Autodesk Inventor part; units mm, degrees
ref_plane "YZ Plane" through (0, 0, 0) normal (1, 0, 0) x (0, 1, 0)
ref_plane "XZ Plane" through (0, 0, 0) normal (0, 1, 0) x (-1, 0, 0)
ref_plane "XY Plane" through (0, 0, 0) normal (0, 0, 1) x (1, 0, 0)
sketch "Эскиз8" plane through (0, 0, 0) normal (1, 0, 0) x (0, 1, 0)
  line L0 (0, 0) -> (10.4, 0)
  line L1 (10.4, 0) -> (10.4, -10.4)
  line L2 (10.4, -10.4) -> (0, -10.4)
  line L3 (0, -10.4) -> (0, 0)
  line L4 (5.2, 0) -> (5.2, 4)
  line L5 (5.2, -10.4) -> (5.2, -14.4)
  circle A0 centre (5.2, 4) radius 1.6
  circle A1 centre (5.2, -14.4) radius 1.6
  line L6 (5.2, 4) -> (7.9, 4)
  line L7 (7.9, 2.4412) -> (5.2, 0.8823)
  line L8 (5.2, 0.8823) -> (2.5, 2.4412)
  line L9 (2.5, 2.4412) -> (2.5, 5.5588)
  line L10 (2.5, 5.5588) -> (5.2, 7.1177)
  line L11 (5.2, 7.1177) -> (7.9, 5.5588)
  line L12 (7.9, 5.5588) -> (7.9, 2.4412)
  line L13 (7.9, -15.9588) -> (5.2, -17.5177)
  line L14 (5.2, -17.5177) -> (2.5, -15.9588)
  line L15 (2.5, -15.9588) -> (2.5, -12.8412)
  line L16 (2.5, -12.8412) -> (5.2, -11.2823)
  line L17 (5.2, -11.2823) -> (7.9, -12.8412)
  line L18 (7.9, -12.8412) -> (7.9, -15.9588)
  circle A2 centre (5.2, 4) radius 5.2
  circle A3 centre (5.2, -14.4) radius 5.2
  line L19 (10.4, 4) -> (10.4, 0)
  line L20 (10.4, -10.4) -> (10.4, -14.4)
  line L21 (0, -14.4) -> (0, -10.4)
  line L22 (0, 4) -> (0, 0)
  line L23 (7.9, 5.5588) -> (7.9, 8.4441)
  line L24 (2.5, 5.5588) -> (2.5, 8.4441)
  line L25 (2.5, -15.9588) -> (2.5, -18.8441)
  line L26 (7.9, -15.9588) -> (7.9, -18.8441)
  line L27 (0, 0) -> (-3, 0)
  line L28 (-3, 0) -> (-3, -10.4)
  line L29 (-3, -10.4) -> (0, -10.4)
  line L30 (0, -10.4) -> (0, 0)
  line L31 (10.4, 0) -> (8.9, 2.5981)
  line L32 (10.4, -10.4) -> (8.9, -12.9981)
  line L33 (10.4, -10.4) -> (13.4, -10.4) construction
  line L34 (8.9, -12.9981) -> (4.4, -10.4)
  line L35 (8.9, 2.5981) -> (4.4, 0)
  line L36 (-3, 0) -> (0.663, 6.5408)
  line L37 (-3, -10.4) -> (0.663, -16.9408)
  line L38 (10.4, 0) -> (12.9981, 1.5)
  line L39 (12.9981, 1.5) -> (9.5707, 6.8173)
  line L40 (10.4, -10.4) -> (12.9981, -11.9)
  line L41 (12.9981, -11.9) -> (9.5707, -17.2173)
  point P0 (7.9, -14.4)
  dimension "d51" = 10.4
  dimension "d52" = 10.4
  dimension "d53" = 4
  dimension "d54" = 4
  dimension "d55" = 3.2
  dimension "d56" = 3.2
  dimension "d57" = 2.7
  dimension "d58" = 3
  dimension "d59" = 3
  dimension "d60" = 3
  dimension "d61" = 120
  dimension "d62" = 3
  dimension "d63" = 3
extrude "Выдавливание6" add sketch "Эскиз8" along normal blind 5 contours L0 A2 L24 L9 L8 L4 L35 | L0 L22 A2 | L4 L7 L12 L23 A2 L31 L35 | L27 L36 A2 L22 | L3 L29 L28 L27 | L31 A2 L19 | L19 A2 L39 L38 | L2 A3 L21 | L21 A3 L37 L29 | L40 L41 A3 L20 | L20 A3 L32 | L2 L34 L5 L16 L15 L25 A3 | A3 L26 L18 L17 L5 L34 L32
sketch "Эскиз9" plane through (0, 0, 0) normal (-1, 0, 0) x (0, 0, 1)
  arc A0 (-18.8441, 2.5) -> (-16.9408, 0.663) centre (-14.4, 5.2) ccw
  circle A1 centre (-14.4, 5.2) radius 5.2
  circle A2 centre (-14.4, 5.2) radius 1.6
  arc A3 (6.5408, 0.663) -> (8.4441, 2.5) centre (4, 5.2) ccw
  circle A4 centre (4, 5.2) radius 5.2
  circle A5 centre (4, 5.2) radius 1.6
  line L0 (2.5981, 8.9) -> (0, 10.4)
  line L1 (0, 10.4) -> (2.5981, 8.9)
  line L2 (0, 4.4) -> (2.5981, 8.9)
  line L3 (2.5981, 8.9) -> (0, 4.4)
  line L4 (0, 0) -> (0, 4.4)
  line L5 (0, 4.4) -> (0, 0)
  line L6 (-10.4, 4.4) -> (-10.4, 0)
  line L7 (0, 0) -> (-10.4, 0)
  line L8 (-10.4, 0) -> (-10.4, 1.8774)
  line L9 (-10.4, 10.4) -> (-12.9981, 8.9)
  line L10 (-11.699, 9.65) -> (-10.4, 10.4)
  line L11 (-11.9, 12.9981) -> (-10.4, 10.4)
  line L12 (-10.4, 10.4) -> (-11.9, 12.9981)
  line L13 (-17.2173, 9.5707) -> (-11.9, 12.9981)
  line L14 (-11.9, 12.9981) -> (-17.2173, 9.5707)
  line L15 (0, 10.4) -> (1.5, 12.9981)
  line L16 (0, 10.4) -> (1.5, 12.9981)
  line L17 (1.5, 12.9981) -> (6.8173, 9.5707)
  line L18 (1.5, 12.9981) -> (6.8173, 9.5707)
  line L19 (0, -3) -> (-10.4, -3)
  line L20 (0, -3) -> (6.5408, 0.663)
  line L21 (6.5408, 0.663) -> (0, -3)
  line L22 (-10.4, -3) -> (-16.9408, 0.663)
  line L23 (-10.4, -3) -> (-16.9408, 0.663)
  line L24 (-10.4, -3) -> (0, -3)
  line L25 (-10.4, 0) -> (0, 0)
  line L26 (0, 0) -> (-10.4, 0)
  line L27 (-10.4, 0) -> (-10.4, 1.8774)
  line L28 (0, 1.8774) -> (0, 0)
  line L29 (-11.699, 9.65) -> (-12.9981, 8.9)
  line L30 (-12.9981, 8.9) -> (-10.4, 4.4)
  line L31 (-10.4, 4.4) -> (-12.9981, 8.9)
  line L32 (-12.9981, 8.9) -> (-10.4, 4.4)
  line L33 (-10.4, 4.4) -> (-10.4, 1.8774)
  line L34 (0, 1.8774) -> (0, 4.4)
  line L35 (2.5981, 8.9) -> (0, 4.4)
  line L36 (1.299, 9.65) -> (2.5981, 8.9)
  point P0 (-18.8441, 2.5)
  point P1 (-16.9408, 0.663)
  point P2 (6.5408, 0.663)
  point P3 (8.4441, 2.5)
  dimension "d66" = 3.2
  dimension "d67" = 3.2
extrude "Выдавливание7" add sketch "Эскиз9" along normal blind 5 contours A1 L9 L30 L6 A0 | A1 L6 L7 L4 A4 L20 L19 L22 | L13 L11 L9 A1 | A4 L4 L2 L0 A3 | L0 L15 L17 A4
sketch "Эскиз10" plane through (5, 0, 0) normal (1, 0, 0) x (0, 0, -1)
  line L0 (-1.5, 12.9981) -> (-6.8173, 9.5707)
  line L1 (0, 10.4) -> (-1.5, 12.9981)
  line L2 (-1.5, 12.9981) -> (0, 10.4)
  line L3 (-2.5981, 8.9) -> (0, 10.4)
  line L4 (0, 10.4) -> (-2.5981, 8.9)
  line L5 (0, 4.4) -> (-2.5981, 8.9)
  line L6 (-2.5981, 8.9) -> (0, 4.4)
  line L7 (0, 0) -> (0, 4.4)
  line L8 (0, 4.4) -> (0, 0)
  line L9 (10.4, 0) -> (0, 0)
  line L10 (0, 0) -> (10.4, 0)
  line L11 (10.4, 4.4) -> (10.4, 0)
  line L12 (10.4, 0) -> (10.4, 4.4)
  line L13 (10.4, 10.4) -> (12.9981, 8.9)
  line L14 (10.4, 4.4) -> (12.9981, 8.9)
  line L15 (12.9981, 8.9) -> (10.4, 10.4)
  line L16 (11.9, 12.9981) -> (10.4, 10.4)
  line L17 (10.4, 10.4) -> (11.9, 12.9981)
  line L18 (17.2173, 9.5707) -> (11.9, 12.9981)
  line L19 (11.9, 12.9981) -> (17.2173, 9.5707)
  line L20 (17.2173, 9.5707) -> (13.6704, -1.1685)
  line L21 (10.4, -3) -> (16.9408, 0.663)
  line L22 (10.4, -3) -> (13.6704, -1.1685)
  line L23 (0, -3) -> (10.4, -3)
  line L24 (-6.5408, 0.663) -> (0, -3)
  line L25 (10.4, -3) -> (0, -3)
  arc A0 (-8.4441, 2.5) -> (-6.5408, 0.663) centre (-4, 5.2) ccw
  line L26 (0, -3) -> (-6.5408, 0.663)
  line L27 (-3.2704, -1.1685) -> (-6.8173, 9.5707)
  line L28 (-6.8173, 9.5707) -> (-1.5, 12.9981)
extrude "Выдавливание8" add sketch "Эскиз10" along normal blind 157.53
sketch "Эскиз13" plane through (162.53, 0, 0) normal (1, 0, 0) x (0, 0, -1)
  line L0 (-6.8173, 9.5707) -> (-1.5, 12.9981)
  line L1 (-1.5, 12.9981) -> (-6.8173, 9.5707)
  line L2 (-6.5408, 0.663) -> (-3.2704, -1.1685)
  line L3 (-6.8173, 9.5707) -> (-3.2704, -1.1685)
  line L4 (-3.2704, -1.1685) -> (0, -3)
  line L5 (10.4, -3) -> (0, -3)
  line L6 (0, -3) -> (10.4, -3)
  line L7 (16.9408, 0.663) -> (10.4, -3)
  line L8 (10.4, -3) -> (13.6704, -1.1685)
  line L9 (13.6704, -1.1685) -> (17.2173, 9.5707)
  line L10 (17.2173, 9.5707) -> (13.6704, -1.1685)
  arc A0 (16.9408, 0.663) -> (17.2173, 9.5707) centre (14.4, 5.2) ccw
  line L11 (17.2173, 9.5707) -> (11.9, 12.9981)
  line L12 (17.2173, 9.5707) -> (11.9, 12.9981)
  line L13 (11.9, 12.9981) -> (10.4, 10.4)
  line L14 (11.9, 12.9981) -> (10.4, 10.4)
  line L15 (10.4, 10.4) -> (12.9981, 8.9)
  line L16 (10.4, 10.4) -> (12.9981, 8.9)
  line L17 (12.9981, 8.9) -> (10.4, 4.4)
  line L18 (10.4, 4.4) -> (12.9981, 8.9)
  line L19 (0, 0) -> (10.4, 0)
  line L20 (10.4, 4.4) -> (10.4, 0)
  line L21 (10.4, 0) -> (0, 0)
  line L22 (0, 4.4) -> (0, 0)
  line L23 (0, 0) -> (0, 4.4)
  line L24 (0, 10.4) -> (-2.5981, 8.9)
  line L25 (0, 4.4) -> (-2.5981, 8.9)
  line L26 (-2.5981, 8.9) -> (0, 10.4)
  line L27 (-1.5, 12.9981) -> (0, 10.4)
  line L28 (0, 10.4) -> (-1.5, 12.9981)
  line L29 (-1.5, 12.9981) -> (11.9, 12.9981)
  line L30 (11.9, 12.9981) -> (11.9, 16.9981)
  line L31 (-1.5, 16.9981) -> (-1.5, 12.9981)
  line L32 (-1.5, 16.9981) -> (0, 16.9981)
  line L33 (0, 20.9981) -> (0, 22.9981)
  line L34 (-1, 23.9981) -> (-0.6923, 23.9981)
  line L35 (-1.5, 21.2778) -> (-1.5, 16.9981)
  line L36 (11.9, 16.9981) -> (10.4, 16.9981)
  line L37 (10.4, 20.9981) -> (10.4, 22.9981)
  line L38 (11.4, 23.9981) -> (11.0923, 23.9981)
  line L39 (11.9, 21.2778) -> (11.9, 16.9981)
  line L40 (-1.5, 23.9981) -> (-1.5, 22.4981)
  line L41 (-6.8173, 9.5707) -> (-3.2704, -1.1685)
  arc A1 (-2.3689, 21.6153) -> (-6.8173, 9.5707) centre (10.1732, 10.1395) ccw
  arc A2 (17.2173, 9.5707) -> (12.7689, 21.6153) centre (0.2268, 10.1395) ccw
  line L42 (11.9, 12.9981) -> (19.7387, 7.9454)
  line L43 (-1.5, 12.9981) -> (-9.3387, 7.9454)
  arc A3 (-2.1057, 23.413) -> (-9.3387, 7.9454) centre (15.5626, 5.726) ccw
  arc A4 (19.7387, 7.9454) -> (12.5057, 23.413) centre (-5.1626, 5.726) ccw
  line L44 (13.6704, -1.1685) -> (16.2685, -2.6685)
  line L45 (13.6704, -1.1685) -> (16.6704, -1.1685) construction
  line L46 (-3.2704, -1.1685) -> (-5.8685, -2.6685)
  line L47 (-3.2704, -1.1685) -> (-0.2704, -1.1685) construction
  line L48 (0, -3) -> (-6.5408, 0.663)
  line L49 (0, -3) -> (-3.7158, -6.3971)
  line L50 (10.4, -3) -> (14.1158, -6.3971)
  spline S0 degree 2 poles (-1.6495, -2.0762) (-2.6908, -8.8998) (-6.9021, -5.2438) knots 0 0 0 1 1 1
  spline S1 degree 2 poles (12.0352, -2.0842) (13.0969, -8.8932) (17.2999, -5.2483) knots 0 0 0 1 1 1
  arc A5 (-9.3387, 7.9454) -> (-6.9021, -5.2438) centre (15.5626, 5.726) ccw
  arc A6 (17.2999, -5.2483) -> (19.7387, 7.9454) centre (-5.1626, 5.726) ccw
  arc A7 (12.7689, 21.6153) -> (11.9, 21.2778) centre (12.4, 21.2778) ccw
  arc A8 (-1.5, 21.2778) -> (-2.3689, 21.6153) centre (-2, 21.2778) ccw
  arc A9 (-0.6923, 23.9981) -> (-2.1057, 23.413) centre (-0.6923, 21.9981) ccw
  arc A10 (12.5057, 23.413) -> (11.0923, 23.9981) centre (11.0923, 21.9981) ccw
  arc A11 (11.4, 23.9981) -> (10.4, 22.9981) centre (11.4, 22.9981) ccw
  arc A12 (0, 22.9981) -> (-1, 23.9981) centre (-1, 22.9981) ccw
  line L51 (1, 19.9981) -> (9.4, 19.9981)
  line L52 (10.4, 16.9981) -> (9.687, 16.9981)
  line L53 (9.687, 16.9981) -> (0, 16.9981)
  arc A13 (0, 20.9981) -> (1, 19.9981) centre (1, 20.9981) ccw
  arc A14 (9.4, 19.9981) -> (10.4, 20.9981) centre (9.4, 20.9981) ccw
  point P0 (0, 23.9981)
  point P1 (10.4, 23.9981)
  point P2 (11.9, 23.9981)
  point P3 (11.9, 22.4981)
  point P4 (0, 19.9981)
  point P5 (10.4, 19.9981)
  point P6 (-6.9021, -5.2438)
  point P7 (-2.7015, -5.4698)
  point P8 (-1.6495, -2.0762)
  point P9 (12.0352, -2.0842)
  point P10 (13.0907, -5.4599)
  point P11 (11.2726, 23.9899)
  point P12 (-0.8726, 23.9899)
  dimension "d78" = 4
  dimension "d80" = 1.5
  dimension "d81" = 1.5
  dimension "d82" = 17
  dimension "d83" = 17
  dimension "d85" = 9.326
  dimension "d86" = 9.326
  dimension "d87" = 25
  dimension "d88" = 25
  dimension "d89" = 3
  dimension "d90" = 30
  dimension "d91" = 3
  dimension "d92" = 150
  dimension "d94" = 0.5
  dimension "d95" = 2
  dimension "d96" = 1
  dimension "d99" = 1
extrude "Выдавливание10" add sketch "Эскиз13" along normal blind 10 contours L43 A3 A9 A12 L33 A13 L51 A14 L37 A11 A10 A4 L42 A2 A7 L39 L36 L52 L53 L32 L35 A8 A1 | L3 L4 S0 L49 A5 L43 | A0 L7 L9 | L42 A6 S1 L50 L7 A0 | S0 L49 | L50 S1
sketch "Эскиз15" plane through (172.53, 0, 0) normal (1, 0, 0) x (0, 0, -1)
  arc A0 (-8.4441, 2.5) -> (-6.5408, 0.663) centre (-4, 5.2) ccw
  arc A1 (-2.1057, 23.413) -> (-6.9021, -5.2438) centre (15.5626, 5.726) ccw
  spline S0 degree 2 poles (-1.6495, -2.0762) (-9.2024, -10.4533) (-8.4441, 2.5) knots 0 0 0 1 1 1
  line L0 (10.4, -3) -> (12.0352, -2.0842)
  line L1 (18.8441, 2.5) -> (14.882, 2.5)
  arc A2 (17.2999, -5.2483) -> (12.5057, 23.413) centre (-5.1626, 5.726) ccw
  spline S1 degree 2 poles (12.0352, -2.0842) (19.6046, -10.4586) (18.8441, 2.5) knots 0 0 0 1 1 1
  line L2 (18.6354, -3) -> (19.4948, 1.6016)
  line L3 (-8.235, -3) -> (-9.0948, 1.6016)
  line L4 (-1.6495, -2.0762) -> (-3.2704, -1.1685)
  spline S2 degree 2 poles (-1.6495, -2.0762) (-2.6908, -8.8998) (-6.9021, -5.2438) knots 0 0 0 1 1 1
  spline S3 degree 2 poles (12.0352, -2.0842) (13.0969, -8.8932) (17.2999, -5.2483) knots 0 0 0 1 1 1
  point P0 (0, 0)
  point P1 (-3.7158, -6.3971)
  point P2 (14.1158, -6.3971)
extrude "Выдавливание11" cut sketch "Эскиз15" against normal blind 10
sketch "Эскиз16" plane through (172.53, 0, 0) normal (1, 0, 0) x (0, 0, -1)
  line L0 (-1.6495, -2.0762) -> (-3.2704, -1.1685)
  line L1 (-2.4412, 2.5) -> (-8.4441, 2.5)
  arc A0 (-2.1057, 23.413) -> (-6.9021, -5.2438) centre (15.5626, 5.726) ccw
  spline S0 degree 2 poles (-1.6495, -2.0762) (-9.2024, -10.4533) (-8.4441, 2.5) knots 0 0 0 1 1 1
  line L2 (13.6704, -1.1685) -> (12.0352, -2.0842)
  arc A1 (16.9408, 0.663) -> (18.8441, 2.5) centre (14.4, 5.2) ccw
  arc A2 (17.2999, -5.2483) -> (12.5057, 23.413) centre (-5.1626, 5.726) ccw
  spline S1 degree 2 poles (12.0352, -2.0842) (19.6046, -10.4586) (18.8441, 2.5) knots 0 0 0 1 1 1
  line L3 (-1.6495, -2.0762) -> (0, -3)
  line L4 (-1.6495, -2.0762) -> (-8.4702, -1.1606)
  line L5 (12.0352, -2.0842) -> (18.8706, -1.1592)
  line L6 (-8.235, -3) -> (-9.0071, 1.1077)
  line L7 (18.6354, -3) -> (19.4075, 1.1099)
  point P0 (0, 0)
  point P1 (18.7195, -2.5523)
  point P2 (-8.319, -2.5532)
extrude "Выдавливание12" add sketch "Эскиз16" against normal blind 10
sketch "Эскиз17" plane through (-5, 0, 0) normal (-1, 0, 0) x (0, 0, 1)
  line L0 (-37.7292, 41.1824) -> (41.3103, 41.1824)
  line L1 (41.3103, 41.1824) -> (41.3103, -34.7876)
  line L2 (41.3103, -34.7876) -> (-37.7292, -34.7876)
  line L3 (-37.7292, -34.7876) -> (-37.7292, 41.1824)
  point P0 (0, 0)
extrude "Выдавливание13" cut sketch "Эскиз17" against normal blind 147.53
sketch "Эскиз18" plane through (172.53, 0, 0) normal (1, 0, 0) x (0, 0, -1)
  line L0 (-31.4647, -11.5956) -> (67.799, -11.5956)
  line L1 (67.799, -11.5956) -> (67.799, 38.6102)
  line L2 (67.799, 38.6102) -> (-31.4647, 38.6102)
  line L3 (-31.4647, 38.6102) -> (-31.4647, -11.5956)
  point P0 (0, 0)
extrude "Выдавливание14" cut sketch "Эскиз18" against normal blind 10
properties part number "защёлка_выдача"
Verification items for the finished model (mm, model axes). A direction names the side the tool comes from. Coordinates: 2 decimals unless noted, no trailing zeros. Write each loop counter-clockwise with the first axis right and the second up, starting at its lowest first coordinate (ties: lowest second). Pieces come first, ordered by that corner, then holes. Notation, with made-up numbers: (35.25, 42.25) - (70.25, 42.25) arc R23 cw to (70.25, 78.25) - close; hole circle Ø9 at (34, -31.5). An arc over 180 degrees is marked (long way). Answer as a JSON object with one key per item and string values.
(1) Cross-section at B-B on x = 160.75. Record the cut outline in (y, z).
Report:
{"outline": "(-3, -10.4) - (-1.17, -13.67) - (9.57, -17.22) - (13, -11.9) - (10.4, -10.4) - (8.9, -13) - (4.4, -10.4) - (0, -10.4) - (0, 0) - (4.4, 0) - (8.9, 2.6) - (10.4, 0) - (13, 1.5) - (9.57, 6.82) - (-1.17, 3.27) - (-3, 0) - close"}
(2) Cross-section at C-C on z = -7.75. Record the cut outline in (x, y), plus the area to 3 significant figures.
Report:
{"outline": "(142.53, -3) - (162.53, -3) - (162.53, 0) - (142.53, 0) - close", "area": "60.0 mm^2"}
(3) Tool access check on faces 1 (the flat face through (152.39, 4.28, -15.47)), 2 (the flat face through (152.39, 11.72, -11.16)), 3 (the flat face through (152.39, 9.64, 1.32)). Record the directions out of +Z, -Z, +X, -X, +Y, -Y that give a thin tool (end or side, any length) a straight path to the whole face; none if there is none.
Report:
{"face 1": "-Z, +X, -X, -Y", "face 2": "+X, -X, +Y", "face 3": "+X, -X"}
(4) Cross-section at A-A on y = 10.75. Record the cut outline in (x, z).
Report:
{"outline": "(142.53, -15.39) - (162.53, -15.39) - (162.53, -10.6) - (142.53, -10.6) - close; (142.53, 0.2) - (162.53, 0.2) - (162.53, 4.99) - (142.53, 4.99) - close"}
(5) Thickness scan on line 1 along Y through (x, z) = (161.5, -10); line 2 along Z through (x, y) = (160.75, 6); line 3 along Z through (x, y) = (150.75, 5.5). Record the ranges inside material, lowest first.
Report:
{"line 1": "-3 to 0", "line 2": "-16.04 to -11.32, 0.92 to 5.64", "line 3": "-15.87 to -11.04, 0.64 to 5.47"}
(6) Gauge pin test, flat ends, axial feed: pin 1 Ø5 at (x, y) = (156.5, 1.5) entering from +Z; pin 2 Ø8.5 at (x, z) = (156.5, -3) entering from +Y; pin 3 Ø1 at (x, y) = (157.5, 7.5) entering from -Z. Record the tip position at first contact, or that the pin passes through.
Report:
{"pin 1": "z = 4.98", "pin 2": "y = 12.57", "pin 3": "z = -16.7"}
(7) Cross-section at D-D on y = 2.5. Record the cut outline in (x, z), plus the area to 3 significant figures.
Report:
{"outline": "(142.53, -14.88) - (162.53, -14.88) - (162.53, -10.4) - (142.53, -10.4) - close; (142.53, 0) - (162.53, 0) - (162.53, 4.48) - (142.53, 4.48) - close", "area": "179 mm^2"}
(8) Mould release check, pull along Z, two halves, no side actions. Record for faces 4 (the flat face through (162.53, -0.2, -5)), 5 (the flat face through (152, 11, -15)), 6 (the flat face through (152.39, 6.62, -11.68)), 7 (the flat face through (152.39, -2.07, 1.66)): pulls with the +Z half, pulls with the -Z half, needs draft (parallel to the pull), parting line crosses it, or undercut.
Report:
{"face 4": "needs draft", "face 5": "pulls with the -Z half", "face 6": "undercut", "face 7": "pulls with the +Z half"}
